Verification items for the finished model (mm, model axes). Give positions to 0.01 mm unless a question says otherwise; leave off trailing zeros. Write each loop counter-clockwise with the first axis right and the second up, starting at its lowest first coordinate (ties: lowest second). Pieces come first, ordered by that corner, then holes. Notation, with made-up numbers: (36.5, 77.5) -> (53.5, 77.5) arc R19 ccw to (53.5, 87.5) -> close; hole circle Ø6 at (66, 1). An arc over 180 degrees is marked (long way). Write item = value, one per line.
from build123d import *

# Parameters (mm, degrees)
F1_DEPTH = 3.175
F2_R     = 3.259298
F2_R_2   = 1.623439
F3_DEPTH = 3.175


with BuildPart() as f1:
    # F0 (on Top) → F1 (new body)
    with BuildSketch(Plane.XY):
        Polygon((116.863699, 10.095269), (-92.469156, 10.095269), (-108.635934, 6.920269), (116.863699, 6.920269), align=None)
    extrude(amount=F1_DEPTH)

    # F2 (on Top) → F3 (join)
    with BuildSketch(Plane.XY):
        with Locations((119.482264, 8.955535)):
            Circle(F2_R)
        with Locations((119.482264, 8.955535)):
            Circle(F2_R_2, mode=Mode.SUBTRACT)
    extrude(amount=F3_DEPTH)


solid = f1.part
Item 1: Sectioned sample at B-B on x = 24. Record the cut outline in (y, z) (3 decimals), then the cut area to 3 significant figures.
Response values:
outline = (6.92, 0) -> (10.095, 0) -> (10.095, 3.175) -> (6.92, 3.175) -> close
area = 10.1 mm^2
Item 2: Go/stop test with flat-tipped pins: P1, Ø1.5, axis at x = 90, y = 11, coming from the -Z side; P2, Ø1.6, axis at x = 46, z = 2, coming from the +Y side; P3, Ø1, axis at x = -49, y = 8, coming from the -Z side. Record where each tip stops, or that it passes through.
Response values:
P1 = through
P2 = 10.1
P3 = 0
Item 3: Sectioned sample at A-A on z = 1.65. Record the cut outline in (x, y).
Response values:
outline = (-108.64, 6.92) -> (116.86, 6.92) -> (116.86, 7.01) arc R3.26 ccw (long way) to (116.43, 10.1) -> (-92.47, 10.1) -> close; hole circle Ø3.25 at (119.48, 8.96)
Item 4: Material ranges on line 1 (Y direction, x = 49, z = 2.9); line 2 (X direction, y = 6.75, z = 1.55); line 3 (X direction, y = 10.75, z = 0.2), recorded low to high.
Response values:
line_1 = 6.92 to 10.1
line_2 = 117.08 to 121.88
line_3 = 116.76 to 122.2
